Input: part model. Units: mm. Frame: model coordinates. A direction names the side the tool comes from. Give positions to 0.01 mm unless a question says otherwise; leave off trailing zeros. Loops run counter-clockwise (first coordinate to the right, second up) from the corner with the lowest first, then second, coordinate; pieces in that order, holes last. Notation, with made-up numbers: (5, 17) -> (49, 17) arc R20 ccw to (49, 36) -> close; hole circle Ø3 at (72, 87). An arc over 180 degrees is marked (long way). Answer as a JSON object with one key per item and string values.
Solid Edge part; units mm, degrees
sketch "Sketch1" plane through (0, 0, 0) normal (0, 0, 1) x (1, 0, 0)
  line L0 (-6.7, 40.3) -> (-6.7, 24)
  line L1 (-6.7, 24) -> (-6.7, 21)
  line L2 (-6.7, 21) -> (-6.7, -11.9391)
  line L3 (-6.7, -11.9391) -> (-6.7, -13.8712)
  line L4 (-6.7, -13.8712) -> (-6.7, -33.0644)
  line L5 (-6.7, -33.0644) -> (-6.7, -36.9)
  line L6 (-6.7, -36.9) -> (-6.7, -42.5)
  line L7 (-6.7, -42.5) -> (7.3, -42.5)
  line L8 (7.3, -42.5) -> (7.3, 21)
  line L9 (7.3, 21) -> (7.3, 24)
  line L10 (7.3, 24) -> (7.3, 40.3)
  line L11 (7.3, 40.3) -> (-6.7, 40.3)
extrude "Protrusion1" add sketch "Sketch1" along normal blind 2.8
sketch "Sketch2" plane through (0, 0, 0) normal (0, 0, 1) x (1, 0, 0)
  line L0 (-6.7, -13.8712) -> (6.9017, -13.2191)
  arc A0 (6.9017, -13.2191) -> (6.8854, -12.4995) centre (6.8845, -12.8595) ccw
  arc A1 (6.8854, -12.4995) -> (-6.7, -11.9391) centre (7.3, 162.5) cw
  line L1 (-6.7, -11.9391) -> (-6.7, -13.8712)
  line L2 (-6.7, -36.9) -> (5.8131, -36.9)
  arc A2 (5.8659, -36.5071) -> (5.8131, -36.9) centre (5.8131, -36.7) cw
  line L3 (-6.7, -33.0644) -> (5.8659, -36.5071)
  line L4 (-6.7, -33.0644) -> (-6.7, -36.9)
extrude "ExtrudedProtrusion_2" add sketch "Sketch2" along normal blind 8.5
sketch "Sketch3" plane through (0, 0, 0) normal (0, 0, 1) x (1, 0, 0)
  line L0 (7.3, 21) -> (-6.7, 21)
  line L1 (-6.7, 24) -> (-6.7, 21)
  line L2 (7.3, 24) -> (-6.7, 24)
  line L3 (7.3, 21) -> (7.3, 24)
extrude "ExtrudedProtrusion_3" add sketch "Sketch3" along normal blind 20
fillet "Round_1" radius 7 2 edges at (7.3, 22.5, 20) (-6.7, 22.5, 20)
fillet "Round_2" radius 0.5 2 edges at (0.1009, -13.5452, 8.5) (-0.417, -34.7857, 8.5)
sketch "Sketch4" plane through (0, 21, 11.4) normal (0, -1, 0) x (1, 0, 0)
  circle A0 centre (0, 3.1) radius 1.8
extrude "ExtrudedCutout_1" cut sketch "Sketch4" against normal blind 3
chamfer "Chamfer_1" distance 2 angle 45 2 edges at (0.3, 21, 2.8) (0.3, 24, 2.8)
Q1. Ray query, line 1 along Z through (x, y) = (0, 22.65); line 2 along Y through (x, z) = (-4.25, 4); line 3 along Y through (x, z) = (-3.75, 3.75). Return the intervals inside material, ascending.
Evaluation:
{"line 1": "z = 0 to 12.7, 16.3 to 19.99", "line 2": "y = -36.9 to -33.74, -13.75 to -12.12, 20.2 to 24.8", "line 3": "y = -36.9 to -33.87, -13.73 to -12.15, 19.95 to 25.05"}
Q2. Access query for faces 4 (the cylindrical face through (-0.234, 22.479, 16.285)), 5 (the cylindrical face through (-0.45, -34.933, 8.357)), 6 (the flat face through (0, 21, 12)). Directions: +Z, -Z, +X, -X, +Y, -Y. A direction counts if a zero-diameter tool reaches every point of the face in a straight line with its end or side. Return the directions, or none.
Evaluation:
{"face 4": "+Y, -Y", "face 5": "+Z, +X", "face 6": "+Z, +X, -X"}
Q3. Draft query along Y for faces 1 (the flat face through (0, 24, 12)), 2 (the flat face through (-1.4, -12.6, 8.5)), 3 (the flat face through (-0.51, -34.76, 5.36)). Return one class per face: +Y half, -Y half, draft (parallel to the pull), parting line (faces both ways), or undercut.
Evaluation:
{"face 1": "+Y half", "face 2": "draft", "face 3": "undercut"}
Q4. Pin query (flat end, axial travel): pin 1 (4.5 mm diameter, centred on x = 1, z = 6, fed in from -Y); pin 2 (4 mm diameter, centred on x = -1.5, y = -13, fed in from +Z); pin 3 (4 mm diameter, centred on x = 0, z = 13, fed in from -Y). Return the tip coordinate at first contact, or that it passes through.
Evaluation:
{"pin 1": "stops at y = -36.9", "pin 2": "stops at z = 8.5", "pin 3": "stops at y = 21"}
Q5. Section C-C, the plane z = 17.75. Return the cut outline in (x, y), then the cut area to 3 significant figures.
Evaluation:
{"outline": "(-4.84, 21) -> (5.44, 21) -> (5.44, 24) -> (-4.84, 24) -> close", "area": "30.9 mm2"}
Q6. Section A-A, the plane z = 14.5. Return the cut outline in (x, y).
Evaluation:
{"outline": "(-6.54, 21) -> (-1.8, 21) -> (-1.8, 24) -> (-6.54, 24) -> close; (1.8, 21) -> (7.14, 21) -> (7.14, 24) -> (1.8, 24) -> close"}
Q7. Section B-B, the plane y = 30. Return the cut outline in (x, z), then the cut area to 3 significant figures.
Evaluation:
{"outline": "(-6.7, 0) -> (7.3, 0) -> (7.3, 2.8) -> (-6.7, 2.8) -> close", "area": "39.2 mm2"}
